from build123d import *

# Parameters (mm, degrees)
F0_R            = 2.7
F1_DEPTH        = 8
F2_R            = 1
F3_DEPTH        = 11
F3_COPIES_COUNT = 3


# Not quite as in the source:
# - a pattern or mirror of a feature is missing from the dataset's text; its kind, count and spacing are read off the source's solid


with BuildPart() as f1:
    # F0 (on Top) → F1 (new body)
    with BuildSketch(Plane.XY):
        Polygon((57.5, 58.4567147554), (-57.5, 58.4567147554), (-67.5, 41.1362066798), (-10, -58.4567147554), (10, -58.4567147554), (67.5, 41.1362066798), align=None)
        with Locations((0, -41.2879311067)):
            Circle(F0_R, mode=Mode.SUBTRACT)
        with Locations((0, -26.2879311067)):
            Circle(F0_R, mode=Mode.SUBTRACT)
        with Locations((0, -6.2879311067)):
            Circle(F0_R, mode=Mode.SUBTRACT)
        Polygon((-10, 48.4567147554), (-10, -38.4567147554), (-55.9529946162, 41.1362066798), (-51.7264973081, 48.4567147554), align=None, mode=Mode.SUBTRACT)
        with Locations((0, 13.7120688933)):
            Circle(F0_R, mode=Mode.SUBTRACT)
        Polygon((51.7264973081, 48.4567147554), (55.9529946162, 41.1362066798), (10, -38.4567147554), (10, 48.4567147554), align=None, mode=Mode.SUBTRACT)
        with Locations((0, 33.7120688933)):
            Circle(F0_R, mode=Mode.SUBTRACT)
        with Locations((0, 48.7120688933)):
            Circle(F0_R, mode=Mode.SUBTRACT)
    extrude(amount=F1_DEPTH)

    # F2 (on face) → F3 (cut)
    with BuildSketch(Plane(origin=(32.8125, -18.9443057078, 0), x_dir=(0.5, 0.8660254038, 0), z_dir=(0.8660254038, -0.5, 0))):
        with Locations((-10.795, 4)):
            Circle(F2_R)
        with Locations((-0.625, 4)):
            Circle(F2_R)
        with Locations((34.545, 4)):
            Circle(F2_R)
        with Locations((24.375, 4)):
            Circle(F2_R)
    f3 = extrude(amount=-F3_DEPTH, mode=Mode.SUBTRACT)

    # F3_copies: F3 ×3 about axis
    f3_copies_axis = Axis((0, 13.712069, 0), (0, 0, 1))
    for i in range(1, F3_COPIES_COUNT):
        add(f3.rotate(f3_copies_axis, i * 360 / F3_COPIES_COUNT), mode=Mode.SUBTRACT)


solid = f1.part
Geometry check sheet. Reference: the model listing, model coordinates, mm. A direction names the side the tool comes from. Round coordinates to 2 decimals unless told otherwise and drop trailing zeros. Order: outer loops, then holes, each group sorted by start corner. A loop starts at its lowest first (then second) coordinate and runs counter-clockwise, first axis right, second up. Notation, with made-up numbers: (17.25, -29.5) - (74.25, -29.5) arc R13 cw to (74.25, -16.5) - close; hole circle Ø4 at (47.5, 18). An arc over 180 degrees is marked (long way). One line per question, with ' | ' between items. Start each with the question number.
(1) Thickness scan on L1, parallel to Y at x = -21, z = 3.5; L2, parallel to X at y = 42, z = 6.5; L3, parallel to X at y = 26.5, z = 1. Record the ranges inside material, lowest first. Write a range as [from, to].
(2) Sectioned sample at C-C on y = -11. Record the cut outline in (x, z).
(3) Access from +Z, -Z, +X, -X, +Y, -Y to the whole of each face (thin tool, end or side, straight path). Record for faces 3 (the flat face through (-31, 48.457, 4)), 4 (the flat face through (0, -58.457, 4)).
(4) Depth check by flat-ended pin: pin 1 Ø1 at (y, z) = (-30, 5.5) entering from +X; pin 2 Ø4 at (x, z) = (27.5, 3) entering from -Y; pin 3 Ø3 at (x, y) = (0, 13.71) entering from -Z; pin 4 Ø1.6 at (x, z) = (-22.67, 4) entering from -Y. Enter the tip coordinate at first touch or a pass-through.
(5) Release check for a two-part mould opening along Z. For faces 1 (the flat face through (10, 4, 4)), 2 (the cylindrical face through (46.292, 14.264, 4.3)) record: released by +Z, released by -Z, zero draft, split by the parting line, or undercut.
(6) Sectioned sample at A-A on x = 0. Record the cut outline in (y, z), and give its area (3 significant figures).
(7) Sectioned sample at B-B on x = 16.5. Record the cut outline in (y, z).
(8) Sectioned sample at D-D on z = 6.5. Count the separate pieces of the cut face and the enclosed holes in it, and give its area (3 significant figures).
Conclusion:
1) L1: y = [-39.4, -25.59], [-23.59, -19.4], [48.46, 58.46] | L2: x = [-67, -55.45], [-10, 10], [55.45, 67] | L3: x = [-59.05, -47.5], [-10, 10], [47.5, 59.05]
2) outline: (-37.4, 0) - (-25.85, 0) - (-25.85, 8) - (-37.4, 8) - close; (-10, 0) - (10, 0) - (10, 8) - (-10, 8) - close; (25.85, 0) - (37.4, 0) - (37.4, 8) - (25.85, 8) - close
3) face 3: +Z, -Z | face 4: +Z, -Z, +X, -X, -Y
4) pin 1: stops at x = 26.72 | pin 2: stops at y = -31.61 | pin 3: passes through | pin 4: stops at y = -37.9
5) face 1: zero draft | face 2: undercut
6) outline: (-58.46, 0) - (-43.99, 0) - (-43.99, 8) - (-58.46, 8) - close; (-38.59, 0) - (-28.99, 0) - (-28.99, 8) - (-38.59, 8) - close; (-23.59, 0) - (-8.99, 0) - (-8.99, 8) - (-23.59, 8) - close; (-3.59, 0) - (11.01, 0) - (11.01, 8) - (-3.59, 8) - close; (16.41, 0) - (31.01, 0) - (31.01, 8) - (16.41, 8) - close; (36.41, 0) - (46.01, 0) - (46.01, 8) - (36.41, 8) - close; (51.41, 0) - (58.46, 0) - (58.46, 8) - (51.41, 8) - close | area: 676 mm2
7) outline: (-47.2, 0) - (-27.2, 0) - (-27.2, 8) - (-47.2, 8) - close; (48.46, 0) - (58.46, 0) - (58.46, 8) - (48.46, 8) - close
8) separate pieces: 1 | enclosed holes: 8 | area: 5,450 mm2
